Model file for the job. Use its own axes, mm. Round coordinates to 2 decimals unless told otherwise and drop trailing zeros. Order: outer loops, then holes, each group sorted by start corner. A loop starts at its lowest first (then second) coordinate and runs counter-clockwise, first axis right, second up. Notation, with made-up numbers: (74, 5) - (126, 5) arc R31 ccw to (126, 37) - close; hole circle Ø10 at (23.5, -30.5). An arc over 180 degrees is marked (long way). Write item = value, one per line. Start each with the question number.
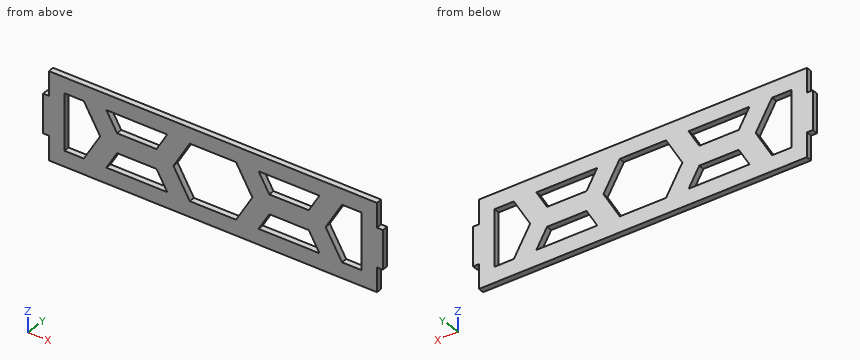
from build123d import *

# Parameters (mm, degrees)
BOSS_EXTRUDE1_DEPTH     = 1.5
CUT_EXTRUDE1_DEPTH      = 2.5
CUT_EXTRUDE1_DEPTH_BACK = 2.5


with BuildPart() as part:
    # Sketch1 → Boss-Extrude1 (new body, symmetric)
    with BuildSketch(Plane(origin=(0, 0, 0), x_dir=(1, 0, 0), z_dir=(0, 1, 0))):
        Polygon((-87, 10), (-87, -10), (-84, -10), (-84, -22.5), (84, -22.5), (84, -10), (87, -10), (87, 10), (84, 10), (84, 22.5), (-84, 22.5), (-84, 10), align=None)
    extrude(amount=BOSS_EXTRUDE1_DEPTH, both=True)

    # Sketch3 → Cut-Extrude1 (cut, two sides)
    with BuildSketch(Plane(origin=(0, 0, 0), x_dir=(1, 0, 0), z_dir=(0, 1, 0))) as cut_extrude1_sk:
        Polygon((-76, -14.5), (-66.106605822, -14.5), (-57.735026919, 0), (-66.106605822, 14.5), (-76, 14.5), align=None)
        Polygon((-20.207259422, 0), (-11.835680518, -14.5), (11.835680518, -14.5), (20.207259422, 0), (11.835680518, 14.5), (-11.835680518, 14.5), align=None)
        Polygon((57.735026919, 0), (66.106605822, -14.5), (76, -14.5), (76, 14.5), (66.106605822, 14.5), align=None)
        Polygon((28.867513459, -5), (23.382685902, -14.5), (54.559600438, -14.5), (49.074772881, -5), align=None)
        Polygon((54.559600438, 14.5), (23.382685902, 14.5), (28.867513459, 5), (49.074772881, 5), align=None)
        Polygon((-49.074772881, -5), (-54.559600438, -14.5), (-23.382685902, -14.5), (-28.867513459, -5), align=None)
        Polygon((-23.382685902, 14.5), (-54.559600438, 14.5), (-49.074772881, 5), (-28.867513459, 5), align=None)
    extrude(amount=CUT_EXTRUDE1_DEPTH, mode=Mode.SUBTRACT)
    extrude(cut_extrude1_sk.sketch, amount=-CUT_EXTRUDE1_DEPTH_BACK, mode=Mode.SUBTRACT)


solid = part.part
Item 1: Saw through at B-B, the plane x = -70.5. Give the cut face in (y, z).
Item 2: Saw through at A-A, the plane x = -36. Give the cut face in (y, z), then the cut area to 3 significant figures.
Item 3: Saw through at D-D, the plane y = -0.75. Give the number of separate pieces and of enclosed holes in the cut face, then the cut area to 3 significant figures.
Item 4: Drop flat-ended pins along their axis: pin 1 (1.5 mm diameter, centred on x = -85.5, y = 0, fed in from -Z); pin 2 (0.9 mm diameter, centred on y = -0.5, z = 17, fed in from +X); pin 3 (10 mm diameter, centred on x = 11.5, z = 1, fed in from +Y); pin 4 (0.9 mm diameter, centred on x = -85.5, y = 0.5, fed in from +Z). Give the stop position or say it passes through.
Item 5: Probe L1, parallel to Z at x = -41, y = -0.4; L2, parallel to X at y = 0.8, z = -9; L3, parallel to X at y = -0.4, z = 9.5. List the from-to ranges inside material, lowest first.
Item 6: Saw through at C-C, the plane z = -2. Give the cut face in (x, y), then the cut area to 3 significant figures.
Check sheet entries:
q1.outline = (-1.5, -22.5) - (1.5, -22.5) - (1.5, -14.5) - (-1.5, -14.5) - close; (-1.5, 14.5) - (1.5, 14.5) - (1.5, 22.5) - (-1.5, 22.5) - close
q2.outline = (-1.5, -22.5) - (1.5, -22.5) - (1.5, -14.5) - (-1.5, -14.5) - close; (-1.5, -5) - (1.5, -5) - (1.5, 5) - (-1.5, 5) - close; (-1.5, 14.5) - (1.5, 14.5) - (1.5, 22.5) - (-1.5, 22.5) - close
q2.area = 78.0 mm2
q3.separate_pieces = 1
q3.enclosed_holes = 7
q3.area = 4,960 mm2
q4.pin_1 = -10
q4.pin_2 = 84
q4.pin_3 = through
q4.pin_4 = 10
q5.L1 = -22.5 to -14.5, -5 to 5, 14.5 to 22.5
q5.L2 = -87 to -76, -62.93 to -51.38, -26.56 to -15.01, 15.01 to 26.56, 51.38 to 62.93, 76 to 87
q5.L3 = -87 to -76, -63.22 to -51.67, -26.27 to -14.72, 14.72 to 26.27, 51.67 to 63.22, 76 to 87
q6.outline = (-87, -1.5) - (-76, -1.5) - (-76, 1.5) - (-87, 1.5) - close; (-58.89, -1.5) - (-19.05, -1.5) - (-19.05, 1.5) - (-58.89, 1.5) - close; (19.05, -1.5) - (58.89, -1.5) - (58.89, 1.5) - (19.05, 1.5) - close; (76, -1.5) - (87, -1.5) - (87, 1.5) - (76, 1.5) - close
q6.area = 305 mm2
